Here's the drawing with two shaded views (mm, measured from the low corner). I have some questions. A direction names the side the tool comes from. Coordinates: 2 decimals unless noted, no trailing zeros. Write each loop counter-clockwise with the first axis right and the second up, starting at its lowest first coordinate (ties: lowest second). Pieces come first, ordered by that corner, then holes. Notation, with made-up numbers: (-36.5, 65) -> (5.5, 65) arc R30 ccw to (5.5, 91) -> close; hole circle Ø4 at (79.5, 79.25). An arc over 180 degrees is marked (long way). Answer in a Markdown table with one row per item. Add a question column.
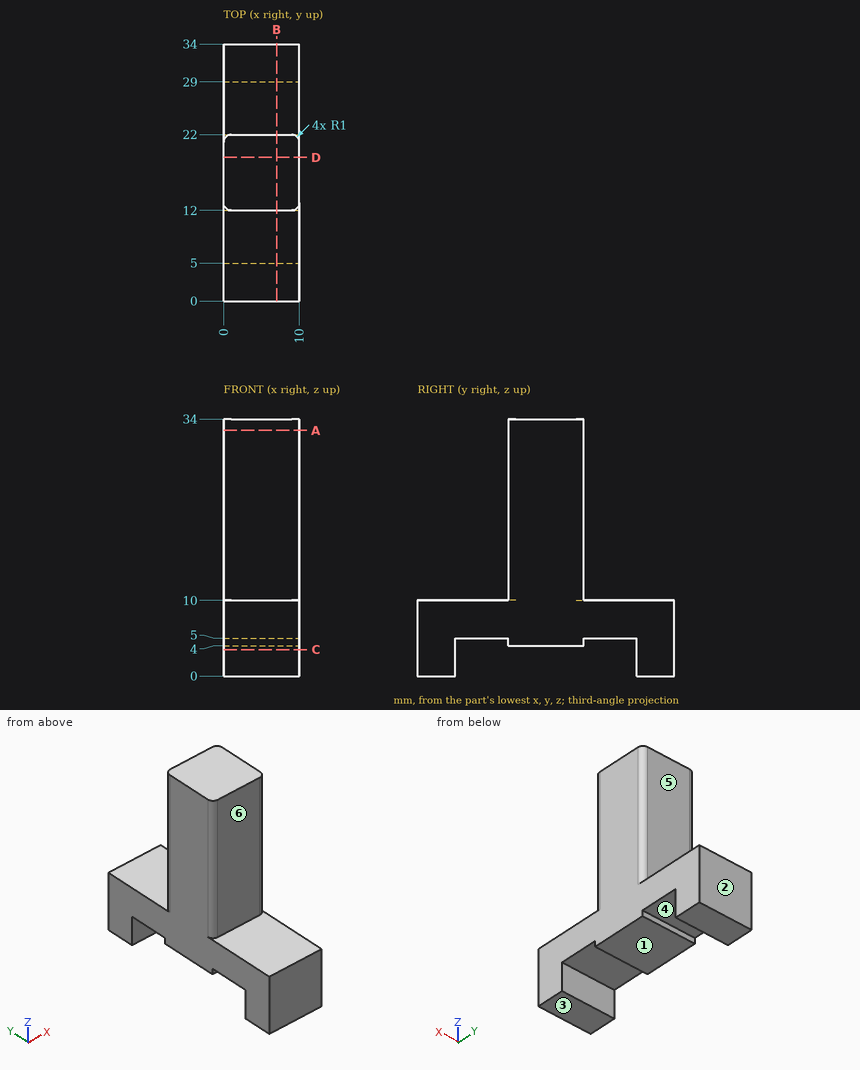
Q1. Imagine slicing it at B-B on x = 7. Please give me the cut outline in (y, z).
Q2. I'm going to push flat-ended pins straight in: P1, Ø2, axis at x = 7, y = 7.5, coming from the -Z side; P2, Ø4, axis at x = 3.5, z = 18, coming from the +Y side; P3, Ø5, axis at x = 2.5, y = 14.5, coming from the -Z side; P4, Ø10, axis at y = 29, z = 19.5, coming from the -X side. Where does each tip first touch, or does it pass through?
Q3. Imagine slicing it at C-C on z = 3.5. Please give me the cut outline in (x, y).
Q4. Imagine slicing it at A-A on z = 32.5. Please give me the cut outline in (x, y), plus the area to 3 significant figures.
Q5. Imagine slicing it at D-D on y = 19. Please give me the cut outline in (x, z).
Q6. I need wall thicknesses on line 1 (Y direction, x = 9.5, z = 3); line 2 (Y direction, x = 1.25, z = 24.5); line 3 (Z direction, x = 8.5, y = 28). Which ranges of each line are inside material? Lowest first, please. Write a range as [from, to].
Q7. For the marked faces 1 and 2, which set-ups out of +Z, -Z, +X, -X, +Y, -Y let a thin tool reach every point of the face, with its end or its side?
Q8. If we mould it in two halves opening along Y, with no side actions, what happens to the marked faces 3, 4, 5 and 6? For each: pulls with the +Y half, pulls with the -Y half, needs draft (parallel to the pull), parting line crosses it, or undercut.
Result sheet:
| question | item | result |
|---|---|---|
| 1 | outline | (0, 0) -> (5, 0) -> (5, 5) -> (12, 5) -> (12, 4) -> (22, 4) -> (22, 5) -> (29, 5) -> (29, 0) -> (34, 0) -> (34, 10) -> (22, 10) -> (22, 34) -> (12, 34) -> (12, 10) -> (0, 10) -> close |
| 2 | P1 | stops at z = 5 |
| 2 | P2 | stops at y = 22 |
| 2 | P3 | stops at z = 4 |
| 2 | P4 | passes through |
| 3 | outline | (0, 0) -> (10, 0) -> (10, 5) -> (0, 5) -> close; (0, 29) -> (10, 29) -> (10, 34) -> (0, 34) -> close |
| 4 | outline | (0, 13) arc R1 ccw to (1, 12) -> (9, 12) arc R1 ccw to (10, 13) -> (10, 21) arc R1 ccw to (9, 22) -> (1, 22) arc R1 ccw to (0, 21) -> close |
| 4 | area | 99.1 mm^2 |
| 5 | outline | (0, 4) -> (10, 4) -> (10, 34) -> (0, 34) -> close |
| 6 | line 1 | y = [0, 5], [29, 34] |
| 6 | line 2 | y = [12, 22] |
| 6 | line 3 | z = [5, 10] |
| 7 | face 1 | -Z, +X, -X |
| 7 | face 2 | +Z, -Z, +X, -X, +Y |
| 8 | face 3 | needs draft |
| 8 | face 4 | undercut |
| 8 | face 5 | pulls with the +Y half |
| 8 | face 6 | pulls with the -Y half |
